Job drawing, mm, ordinate dimensions from the low corner. One solid piece. A direction names the side the tool comes from. Coordinates: 2 decimals unless noted, no trailing zeros. Write each loop counter-clockwise with the first axis right and the second up, starting at its lowest first coordinate (ties: lowest second). Pieces come first, ordered by that corner, then holes.
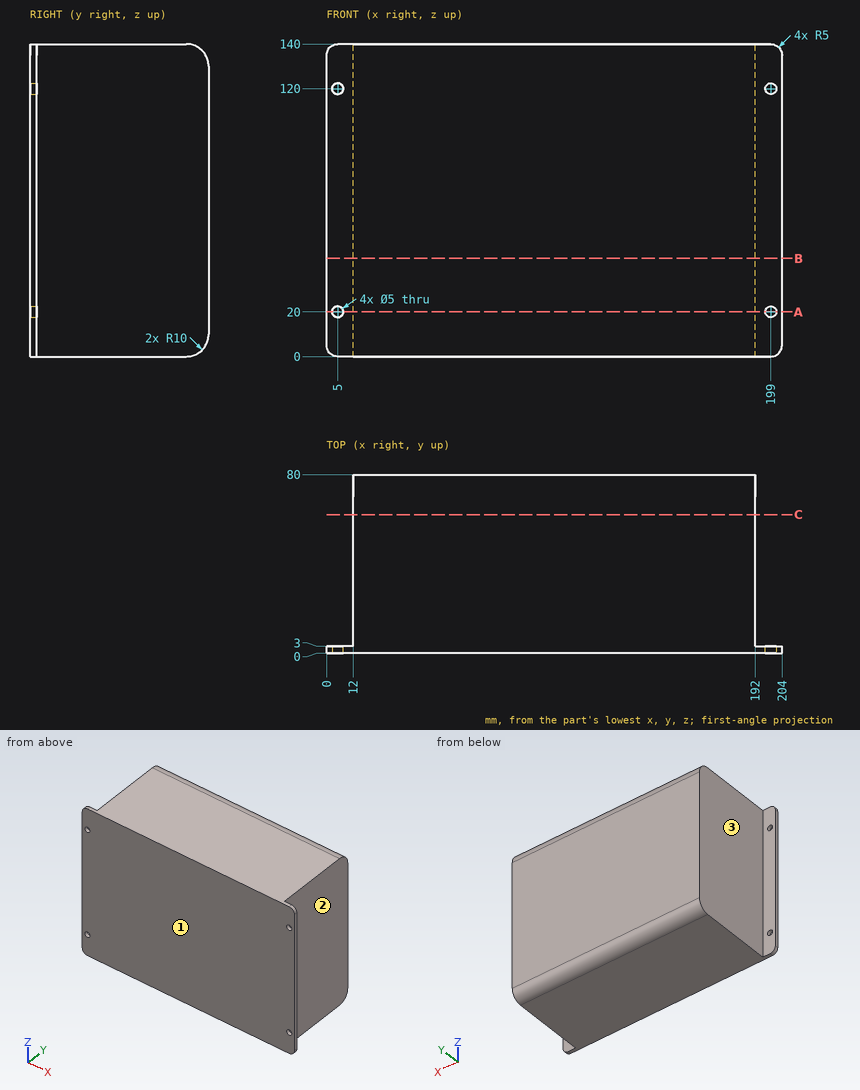
1. Saw through at A-A on z = 20. List the corners of the cut face in (x, y), plus the area to 3 significant figures.
Computed values:
outline: (0, 0) - (2.5, 0) - (2.5, 3) - (0, 3) - close; (7.5, 0) - (196.5, 0) - (196.5, 3) - (192, 3) - (192, 80) - (12, 80) - (12, 3) - (7.5, 3) - close; (201.5, 0) - (204, 0) - (204, 3) - (201.5, 3) - close
area: 14,400 mm2
2. Saw through at B-B on z = 44. List the corners of the cut face in (x, y).
Computed values:
outline: (0, 0) - (204, 0) - (204, 3) - (192, 3) - (192, 80) - (12, 80) - (12, 3) - (0, 3) - close
3. Flat gauge pins, fed straight in: pin 1 (23 mm diameter, centred on y = 32, z = 70.5, fed in from -X); pin 2 (3.5 mm diameter, centred on x = 4, z = 95, fed in from +Y). Where does each tip first touch, or does it go through?
Computed values:
pin 1: stops at x = 12
pin 2: stops at y = 3
4. Saw through at C-C on y = 62. List the corners of the cut face in (x, z).
Computed values:
outline: (12, 0) - (192, 0) - (192, 140) - (12, 140) - close
5. 3-axis set-ups, long thin cutter, end or side, ignore diameter. For the marked faces 1, 2 and 3: which of +Z, -Z, +X, -X, +Y, -Y reach the whole face in a straight line?
Computed values:
face 1: +Z, -Z, +X, -X, -Y
face 2: +Z, -Z, +X, +Y
face 3: +Z, -Z, -X, +Y
6. Probe line 1 along X through (y, z) = (2.3, 120); line 2 along Z through (x, y) = (199, 1.55); line 3 along Y through (x, z) = (193, 62). List the from-to ranges inside material, lowest first.
Computed values:
line 1: x = 0 to 2.5, 7.5 to 196.5, 201.5 to 204
line 2: z = 0 to 17.5, 22.5 to 117.5, 122.5 to 140
line 3: y = 0 to 3
